Verification items for the finished model (mm, model axes). Coordinates: 2 decimals unless noted, no trailing zeros. Order: outer loops, then holes, each group sorted by start corner. A loop starts at its lowest first (then second) coordinate and runs counter-clockwise, first axis right, second up. Notation, with made-up numbers: M 65,-11 L 72,-11 A18 cw 72,23 Z; hole C -8,82.25 d2. An arc over 180 degrees is marked long. Return JSON: item names as keys, results as strings. Group by question number.
Q1. Thickness scan on probe 1 along X at (y, z) = (38, -8); probe 2 along Y at (x, z) = (0, 18); probe 3 along Y at (x, z) = (-9, -1). Record the ranges inside material, lowest first.
Q2. Section check B-B, the plane x = 0. Enter the section's corners in (y, z), then the cut area to 3 significant figures.
Q3. Section check C-C, the plane z = 28. Enter the section's corners in (x, y), then the cut area to 3 significant figures.
Q4. Section check A-A, the plane y = 38.1. Enter the section's corners in (x, z).
Q5. Mould release check, pull along X, two halves, no side actions. Record for faces 1 (the face through (0, 50, -31.75)), 2 (the face through (-25.4, 50, 0)), 3 (the face through (-1.389, 48.677, -0.445)), 4 (the face through (25.4, 50, 0)): pulls with the +X half, pulls with the -X half, needs draft (parallel to the pull), parting line crosses it, or undercut.
Q6. Go/stop test with a flat-tipped pin: pin 1 Ø12 at (x, z) = (9.5, 22) entering from -Y. Record where the tip stops, or that it passes through.
from build123d import *

# Parameters (mm, degrees)
SKETCH1_W               = 50.8
SKETCH1_H               = 63.5
BOSS_EXTRUDE2_DEPTH     = 101.6
CUT_EXTRUDE2_DEPTH      = 110.433918417
CUT_EXTRUDE2_DEPTH_BACK = 110.433918417
SKETCH4_R               = 10.668


with BuildPart() as part:
    # Sketch1 → Boss-Extrude2 (new body)
    with BuildSketch(Plane(origin=(0, 0, 0), x_dir=(1, 0, 0), z_dir=(0, 1, 0))):
        Rectangle(SKETCH1_W, SKETCH1_H)
    extrude(amount=BOSS_EXTRUDE2_DEPTH)

    # Sketch4 → Cut-Extrude2 (cut, two sides: drawn at the far end of the back side and taken through both)
    with BuildSketch(Plane.XY.offset(-CUT_EXTRUDE2_DEPTH_BACK)):
        with Locations((0, 38.1)):
            Circle(SKETCH4_R)
    extrude(amount=CUT_EXTRUDE2_DEPTH + CUT_EXTRUDE2_DEPTH_BACK, mode=Mode.SUBTRACT)


solid = part.part
Numbers:
{
 "1": {"probe 1": "x = -25.4 to -10.67, 10.67 to 25.4", "probe 2": "y = 0 to 27.43, 48.77 to 101.6", "probe 3": "y = 0 to 32.37, 43.83 to 101.6"},
 "2": {"outline": "M 0,-31.75 L 27.43,-31.75 L 27.43,31.75 L 0,31.75 Z; M 48.77,-31.75 L 101.6,-31.75 L 101.6,31.75 L 48.77,31.75 Z", "area": "5,100 mm2"},
 "3": {"outline": "M -25.4,0 L 25.4,0 L 25.4,101.6 L -25.4,101.6 Z; hole C 0,38.1 d21.34", "area": "4,800 mm2"},
 "4": {"outline": "M -25.4,-31.75 L -10.67,-31.75 L -10.67,31.75 L -25.4,31.75 Z; M 10.67,-31.75 L 25.4,-31.75 L 25.4,31.75 L 10.67,31.75 Z"},
 "5": {"face 1": "needs draft", "face 2": "pulls with the -X half", "face 3": "undercut", "face 4": "pulls with the +X half"},
 "6": {"pin 1": "stops at y = 0"}
}
